Input: part model. Units: mm. Frame: model coordinates. Give positions to 0.01 mm unless a question says otherwise; leave off trailing zeros. Loops run counter-clockwise (first coordinate to the right, second up) from the corner with the lowest first, then second, coordinate; pieces in that order, holes last. Notation, with made-up numbers: (18.5, 47.5) - (36.5, 47.5) arc R20 ccw to (36.5, 52.5) - close; hole circle Ø11 at (-35, 8). An arc over 180 degrees is marked (long way). Answer as a JSON object with one key per item and string values.
from build123d import *

# Parameters (mm, degrees)
MODEL_R                 = 1.6
MODEL_R_2               = 2.75
SALIENTE_EXTRUIR1_DEPTH = 3


with BuildPart() as part:
    # Model → Saliente-Extruir1 (new body)
    with BuildSketch(Plane.XY):
        with BuildLine():
            Line((154.018604018, 58.836275918), (79.516105518, 58.836274418))
            ThreePointArc((79.516105518, 58.836274418), (79.162552127, 58.982721028), (79.016105518, 59.336274418))
            Line((79.016105518, 59.336274418), (79.016105518, 64.834297418))
            ThreePointArc((79.016105518, 64.834297418), (78.43031908, 66.248510981), (77.016105518, 66.834297418))
            Line((77.016105518, 66.834297418), (72.69995292, 66.834297418))
            ThreePointArc((72.69995292, 66.834297418), (72.258226513, 66.568557489), (72.286037482, 66.053808542))
            ThreePointArc((72.286037482, 66.053808542), (69.016105518, 59.887946419), (65.746173553, 66.053808542))
            ThreePointArc((65.746173553, 66.053808542), (65.773984522, 66.56855749), (65.332258115, 66.834297418))
            Line((65.332258115, 66.834297418), (61.016105518, 66.834297418))
            ThreePointArc((61.016105518, 66.834297418), (59.601891956, 66.248510981), (59.016105518, 64.834297418))
            Line((59.016105518, 64.834297418), (59.016105518, 59.336277418))
            ThreePointArc((59.016105518, 59.336277418), (58.869658908, 58.982724028), (58.516105518, 58.836277418))
            Line((58.516105518, 58.836277418), (28.843601518, 58.836277418))
            Line((28.843601518, 58.836277418), (23.843601518, 58.836277418))
            ThreePointArc((23.843601518, 58.836277418), (20.308067612, 57.371811324), (18.843601518, 53.836277418))
            Line((18.843601518, 53.836277418), (18.843601518, 19.448682418))
            ThreePointArc((18.843601518, 19.448682418), (20.308068445, 15.91314768), (23.843603874, 14.448682418))
            Line((23.843603874, 14.448682418), (43.108834237, 14.448682418))
            ThreePointArc((43.108834237, 14.448682418), (43.70094804, 14.642828062), (44.063149212, 15.149879929))
            Line((44.063149212, 15.149879929), (45.624053822, 20.135094908))
            ThreePointArc((45.624053822, 20.135094908), (45.986254995, 20.642146775), (46.578368798, 20.836292418))
            Line((46.578368798, 20.836292418), (154.018604018, 20.833862066))
            Line((154.018604018, 20.833862066), (261.458839238, 20.836292418))
            ThreePointArc((261.458839238, 20.836292418), (262.050953041, 20.642146775), (262.413154213, 20.135094908))
            Line((262.413154213, 20.135094908), (263.974058823, 15.149879929))
            ThreePointArc((263.974058823, 15.149879929), (264.336259996, 14.642828062), (264.928373799, 14.448682418))
            Line((264.928373799, 14.448682418), (284.193604162, 14.448682418))
            ThreePointArc((284.193604162, 14.448682418), (287.729139591, 15.91314768), (289.193606518, 19.448682418))
            Line((289.193606518, 19.448682418), (289.193606518, 53.836277418))
            ThreePointArc((289.193606518, 53.836277418), (287.729140424, 57.371811324), (284.193606518, 58.836277418))
            Line((284.193606518, 58.836277418), (279.193606518, 58.836277418))
            Line((279.193606518, 58.836277418), (249.521102518, 58.836277418))
            ThreePointArc((249.521102518, 58.836277418), (249.167549127, 58.982724028), (249.021102518, 59.336277418))
            Line((249.021102518, 59.336277418), (249.021102518, 64.834297418))
            ThreePointArc((249.021102518, 64.834297418), (248.43531608, 66.248510981), (247.021102518, 66.834297418))
            Line((247.021102518, 66.834297418), (242.704949921, 66.834297418))
            ThreePointArc((242.704949921, 66.834297418), (242.263223513, 66.56855749), (242.291034482, 66.053808542))
            ThreePointArc((242.291034482, 66.053808542), (239.021102518, 59.887946419), (235.751170554, 66.053808542))
            ThreePointArc((235.751170554, 66.053808542), (235.778981523, 66.568557489), (235.337255116, 66.834297418))
            Line((235.337255116, 66.834297418), (231.021102518, 66.834297418))
            ThreePointArc((231.021102518, 66.834297418), (229.606888956, 66.248510981), (229.021102518, 64.834297418))
            Line((229.021102518, 64.834297418), (229.021102518, 59.336274418))
            ThreePointArc((229.021102518, 59.336274418), (228.874655908, 58.982721028), (228.521102518, 58.836274418))
            Line((228.521102518, 58.836274418), (154.018604018, 58.836275918))
        make_face()
        with Locations((69.016105518, 53.837946418)):
            Circle(MODEL_R, mode=Mode.SUBTRACT)
        with Locations((154.018604018, 39.835068992)):
            Circle(MODEL_R, mode=Mode.SUBTRACT)
        with Locations((239.021102518, 53.837946418)):
            Circle(MODEL_R, mode=Mode.SUBTRACT)
        with Locations((40.904504018, 31.448682418)):
            Circle(MODEL_R_2, mode=Mode.SUBTRACT)
        with Locations((267.132704018, 31.448682418)):
            Circle(MODEL_R_2, mode=Mode.SUBTRACT)
        Polygon((144.018604018, 39.835068992), (144.018604018, 49.835068992), (149.018604018, 49.835068992), (149.018604018, 29.835068992), (144.018604018, 29.835068992), align=None, mode=Mode.SUBTRACT)
        Polygon((164.018604018, 39.835068992), (164.018604018, 49.835068992), (159.018604018, 49.835068992), (159.018604018, 29.835068992), (164.018604018, 29.835068992), align=None, mode=Mode.SUBTRACT)
    extrude(amount=SALIENTE_EXTRUIR1_DEPTH)


solid = part.part
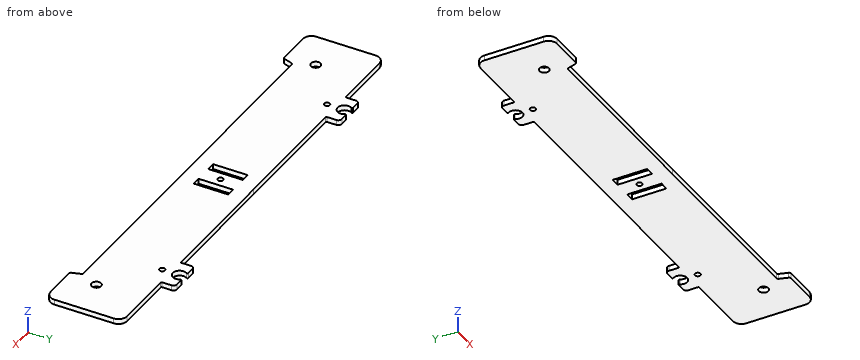
Item 1: Contact query for flat-ended pins moving along their axis: P1, Ø0.9, axis at y = 61, z = 2, coming from the -X side; P2, Ø1.5, axis at x = 190, z = 1.5, coming from the -Y side; P3, Ø1.5, axis at y = 61, z = 2, coming from the +X side; P4, Ø3.5, axis at x = 40.9, y = 31.45, coming from the -Z side. Output: stop coordinate, or through.
Geometry check:
{"P1": "stops at x = 59.02", "P2": "stops at y = 20.83", "P3": "stops at x = 249.02", "P4": "passes through"}
Item 2: Cut plane C-C (x = 255). Return loops of the section in (y, z).
Geometry check:
{"outline": "(20.84, 0) - (58.84, 0) - (58.84, 3) - (20.84, 3) - close"}
Item 3: Cut plane A-A (y = 46.5). Return loops of the section in (x, z), then the cut area to 3 significant figures.
Geometry check:
{"outline": "(18.84, 0) - (144.02, 0) - (144.02, 3) - (18.84, 3) - close; (149.02, 0) - (159.02, 0) - (159.02, 3) - (149.02, 3) - close; (164.02, 0) - (289.19, 0) - (289.19, 3) - (164.02, 3) - close", "area": "781 mm2"}
Item 4: Cut plane B-B (z = 1.5). Give the number of separate pieces and of enclosed holes in the cut face, then the cut area to 3 significant figures.
Geometry check:
{"separate pieces": "1", "enclosed holes": "7", "area": "10,500 mm2"}
Item 5: Material intervals for line 1 (X direction, y = 45, z = 1.35); line 2 (X direction, y = 53.5, z = 0.7) (3 decimals); line 3 (X direction, y = 61, z = 1.6), sorted ascending. Write a range as [from, to].
Geometry check:
{"line 1": "x = [18.84, 144.02], [149.02, 159.02], [164.02, 289.19]", "line 2": "x = [18.844, 67.452], [70.58, 237.457], [240.585, 289.194]", "line 3": "x = [59.02, 66.27], [71.76, 79.02], [229.02, 236.27], [241.77, 249.02]"}
